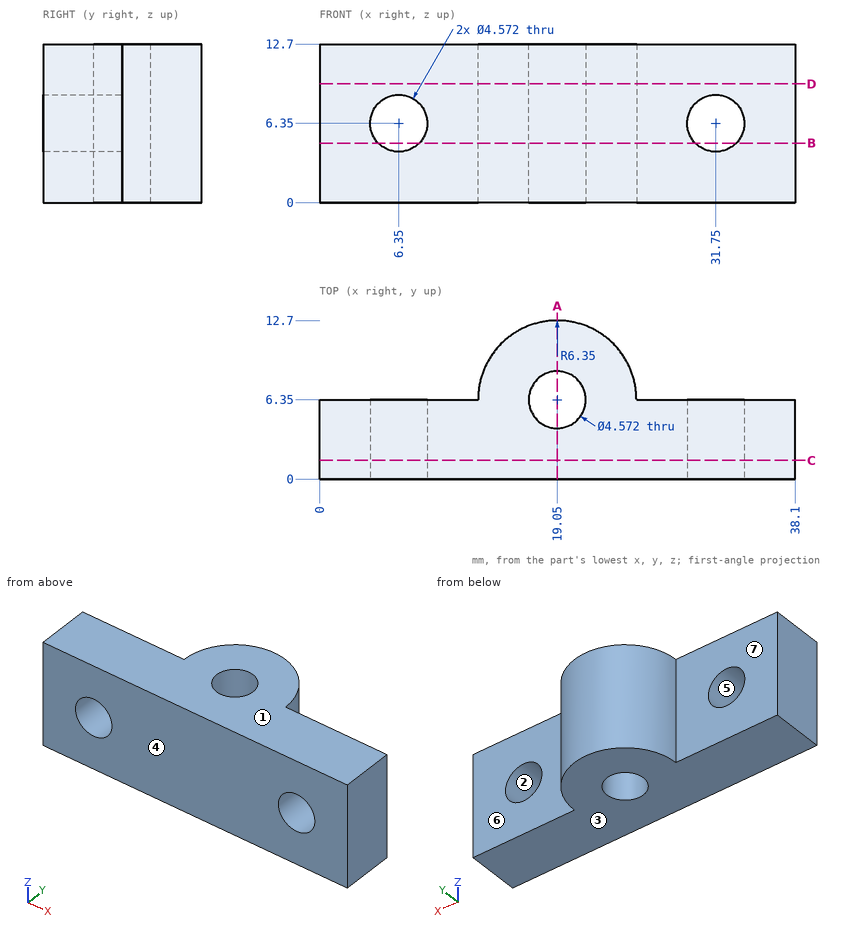
The drawing under review shows one solid part. Ordinate dimensions are in mm from its lowest x, y, z. A direction names the side the tool comes from. Coordinates: 2 decimals unless noted, no trailing zeros. Order: outer loops, then holes, each group sorted by start corner. A loop starts at its lowest first (then second) coordinate and runs counter-clockwise, first axis right, second up. Notation, with made-up numbers: (87.25, -22) -> (92.25, -22) arc R21 ccw to (92.25, -9) -> close; hole circle Ø1 at (29, -34.5). An arc over 180 degrees is marked (long way). Answer as CSV lines item,"result".
Q1. We need section B-B (z = 4.75). State the section outline as (x, y) points.
Model answer:
outline,"(0, 0) -> (4.72, 0) -> (4.72, 6.35) -> (0, 6.35) -> close; (7.98, 0) -> (30.12, 0) -> (30.12, 6.35) -> (25.4, 6.35) arc R6.35 ccw to (12.7, 6.35) -> (7.98, 6.35) -> close; (33.38, 0) -> (38.1, 0) -> (38.1, 6.35) -> (33.38, 6.35) -> close; hole circle Ø4.57 at (19.05, 6.35)"
Q2. For the marked faces 5, 6 and 7, list the 3-axis set-ups (+Z, -Z, +X, -X, +Y, -Y) from which the entire face can be reached by the end or side of a thin tool; tool diameter is ignored.
Model answer:
face 5,"+Y, -Y"
face 6,"+Z, -Z, +X, +Y"
face 7,"+Z, -Z, -X, +Y"
Q3. We need section D-D (z = 9.5). State the section outline as (x, y) points.
Model answer:
outline,"(0, 0) -> (38.1, 0) -> (38.1, 6.35) -> (25.4, 6.35) arc R6.35 ccw to (12.7, 6.35) -> (0, 6.35) -> close; hole circle Ø4.57 at (19.05, 6.35)"
Q4. We need section C-C (y = 1.5). State the section outline as (x, z) points.
Model answer:
outline,"(0, 0) -> (38.1, 0) -> (38.1, 12.7) -> (0, 12.7) -> close; hole circle Ø4.57 at (6.35, 6.35); hole circle Ø4.57 at (31.75, 6.35)"
Q5. Draft analysis for pull direction Z (two halves, no side actions). For the marked faces 1, 2, 3 and 4, state which applies: released by +Z, released by -Z, zero draft, split by the parting line, or undercut.
Model answer:
face 1,"released by +Z"
face 2,"undercut"
face 3,"released by -Z"
face 4,"zero draft"
Q6. Wall thickness on line 1 along X through (y, z) = (4, 6.35); line 2 along X through (y, z) = (4.5, 6.35); line 3 along Y through (x, z) = (9, 8.25): over which ranges is each line inside the solid? List them lowest first. Write a range as [from, to].
Model answer:
line 1,"x = [0, 4.06], [8.64, 29.46], [34.04, 38.1]"
line 2,"x = [0, 4.06], [8.64, 17.71], [20.39, 29.46], [34.04, 38.1]"
line 3,"y = [0, 6.35]"
Q7. Clearance check with flat-ended pins moving along their axes: pin 1 Ø3.5 at (x, z) = (31.75, 6.35) entering from +Y; pin 2 Ø6.5 at (x, z) = (33, 5.5) entering from +Y. State where each tip first meets the part, or that it passes through.
Model answer:
pin 1,"passes through"
pin 2,"stops at y = 6.35"
Q8. We need section A-A (x = 19.05). State the section outline as (y, z) points.
Model answer:
outline,"(0, 0) -> (4.06, 0) -> (4.06, 12.7) -> (0, 12.7) -> close; (8.64, 0) -> (12.7, 0) -> (12.7, 12.7) -> (8.64, 12.7) -> close"
